Source: CAD feature listing. Evaluate the final solid. Frame: model axes, mm. Give positions to 0.01 mm unless a question says otherwise; leave off trailing zeros. Write each loop counter-clockwise with the first axis right and the second up, starting at its lowest first coordinate (ties: lowest second). Pieces come first, ordered by that corner, then holes. Notation, with made-up numbers: (17.5, 34.25) -> (29.5, 34.25) arc R14 cw to (29.5, 46.25) -> close; hole circle Ø8 at (27, -25). An arc over 180 degrees is marked (long way). Write item = value, one per line.
from build123d import *

# Parameters (mm, degrees)
EXTRUDE_1_DEPTH     = 3
SKETCH_2_R          = 4.5
CUT_EXTRUDE_1_DEPTH = 40.736632973
SKETCH_3_R          = 0.8
CUT_EXTRUDE_2_DEPTH = 40.736632973


with BuildPart() as part:
    # Эскиз1 → Бобышка-Вытянуть1 (new body)
    with BuildSketch(Plane.XY):
        with BuildLine():
            Line((4, 0), (25, 0))
            ThreePointArc((25, 0), (27.828427125, 1.171572875), (29, 4))
            Line((29, 4), (29, 23))
            ThreePointArc((29, 23), (27.828427125, 25.828427125), (25, 27))
            Line((25, 27), (4, 27))
            ThreePointArc((4, 27), (1.171572875, 25.828427125), (0, 23))
            Line((0, 23), (0, 4))
            ThreePointArc((0, 4), (1.171572875, 1.171572875), (4, 0))
        make_face()
    extrude(amount=EXTRUDE_1_DEPTH)

    # Эскиз2 → Вырез-Вытянуть1 (cut, through all)
    with BuildSketch(Plane.XY.offset(3)):
        with Locations((14.5, 13.5)):
            Circle(SKETCH_2_R)
    extrude(amount=-CUT_EXTRUDE_1_DEPTH, mode=Mode.SUBTRACT)

    # Эскиз3 → Вырез-Вытянуть2 (cut, through all)
    with BuildSketch(Plane.XY.offset(3)):
        with Locations((3.5, 4)):
            Circle(SKETCH_3_R)
        with Locations((25.5, 4)):
            Circle(SKETCH_3_R)
        with Locations((25.5, 23)):
            Circle(SKETCH_3_R)
        with Locations((3.5, 23)):
            Circle(SKETCH_3_R)
    extrude(amount=-CUT_EXTRUDE_2_DEPTH, mode=Mode.SUBTRACT)


solid = part.part
1) Draft query along X for faces 1 (the cylindrical face through (25.87, 22.29, 1.52)), 2 (the cylindrical face through (1.203, 25.859, 1.479)), 3 (the cylindrical face through (27.859, 25.797, 1.479)). Return one class per face: pulls with the +X half, pulls with the -X half, needs draft (parallel to the pull), parting line crosses it, or undercut.
Computed:
face_1 = undercut
face_2 = pulls with the -X half
face_3 = pulls with the +X half
2) Cut plane C-C (y = 12.25). Return the cut outline in (x, z), then the cut area to 3 significant figures.
Computed:
outline = (0, 0) -> (10.18, 0) -> (10.18, 3) -> (0, 3) -> close; (18.82, 0) -> (29, 0) -> (29, 3) -> (18.82, 3) -> close
area = 61.1 mm²
3) Cut plane D-D (x = 25.5). Return the cut outline in (y, z).
Computed:
outline = (0.03, 0) -> (3.2, 0) -> (3.2, 3) -> (0.03, 3) -> close; (4.8, 0) -> (22.2, 0) -> (22.2, 3) -> (4.8, 3) -> close; (23.8, 0) -> (26.97, 0) -> (26.97, 3) -> (23.8, 3) -> close
4) Material intervals for L1, parallel to Y at x = 3.5, z = 2.1; L2, parallel to Y at x = 10.5, z = 0.7; L3, parallel to Y at x = 13.75, z = 1.1, sorted ascending.
Computed:
L1 = 0.03 to 3.2, 4.8 to 22.2, 23.8 to 26.97
L2 = 0 to 11.44, 15.56 to 27
L3 = 0 to 9.06, 17.94 to 27
5) Cut plane A-A (x = 14.5). Return the cut outline in (y, z).
Computed:
outline = (0, 0) -> (9, 0) -> (9, 3) -> (0, 3) -> close; (18, 0) -> (27, 0) -> (27, 3) -> (18, 3) -> close
6) Cut plane B-B (z = 1.75). Return the cut outline in (x, y).
Computed:
outline = (0, 4) arc R4 ccw to (4, 0) -> (25, 0) arc R4 ccw to (29, 4) -> (29, 23) arc R4 ccw to (25, 27) -> (4, 27) arc R4 ccw to (0, 23) -> close; hole circle Ø1.6 at (3.5, 4); hole circle Ø1.6 at (3.5, 23); hole circle Ø9 at (14.5, 13.5); hole circle Ø1.6 at (25.5, 4); hole circle Ø1.6 at (25.5, 23)
